Could you check a few things on this model? Use its own coordinates, in mm. A direction names the side the tool comes from. Round coordinates to 2 decimals unless told otherwise and drop trailing zeros. Loops run counter-clockwise (first coordinate to the right, second up) from the corner with the lowest first, then second, coordinate; pieces in that order, holes last. Notation, with made-up numbers: M -26,76.25 L -18,76.25 A19 ccw -18,113.25 Z; hole C 44.5,37.25 d3. An arc over 180 degrees is marked long. Return JSON: item names as keys, results as strings. Group by question number.
```python
from build123d import *

# Parameters (mm, degrees)
F2_DEPTH = 25


# Not quite as in the source:
# - a feature names something its author has since deleted; it is built from what else it names


with BuildPart() as f1:
    # F0 (on Front) → F1 (revolve)
    with BuildSketch(Plane.XZ):
        with BuildLine():
            Line((0, 9.9311807901), (0, 10.9311807901))
            Line((0, 10.9311807901), (-3.4236455734, 10.9311807901))
            ThreePointArc((-3.4236455734, 10.9311807901), (-3.9013040029, 10.5789726191), (-4.3789624324, 10.9311807901))
            Line((-4.3789624324, 10.9311807901), (-15.6210375676, 10.9311807901))
            ThreePointArc((-15.6210375676, 10.9311807901), (-16.0986959971, 10.5789726191), (-16.5763544266, 10.9311807901))
            Line((-16.5763544266, 10.9311807901), (-20, 10.9311807901))
            Line((-20, 10.9311807901), (-20, 9.9311807901))
            Line((-20, 9.9311807901), (-19, 9.9311807901))
            Line((-19, 9.9311807901), (-19, 7.4311807901))
            Line((-19, 7.4311807901), (-18.118519783, 7.4311807901))
            Line((-18.118519783, 7.4311807901), (-18.118519783, 3.4311807901))
            Line((-18.118519783, 3.4311807901), (-1.881480217, 3.4311807901))
            Line((-1.881480217, 3.4311807901), (-1.881480217, 7.4311807901))
            Line((-1.881480217, 7.4311807901), (-1, 7.4311807901))
            Line((-1, 7.4311807901), (-1, 9.9311807901))
            Line((-1, 9.9311807901), (0, 9.9311807901))
        make_face()
    revolve(axis=Axis((-10, 0, 3.4311807901), (-1, 0, 0)))

    # F2 (cut): a face of the model
    f2_faces = [f1.faces().sort_by_distance(p)[0] for p in [
        (-18.118519783, 0, 3.4311807901),
    ]]
    extrude(f2_faces, amount=-F2_DEPTH, mode=Mode.SUBTRACT)


solid = f1.part
```
1. I'm going to push flat-ended pins straight in: pin 1 Ø4 at (y, z) = (1, 5.5) entering from +X; pin 2 Ø6 at (x, y) = (-9.5, -5) entering from -Z; pin 3 Ø3 at (x, y) = (-15.5, -2) entering from -Z. Where does each tip first touch, or does it pass through?
2. We'd pull the mould along Y, two halves only. Please class faces 4 (the face through (-20, 7, 3)), 5 (the face through (-10.08, -2.87, 10.36)), 6 (the face through (-1, -4.2, 3.5)): +Y half, -Y half, draft (parallel to the pull), parting line (faces both ways), or undercut.
3. If we section it at A-A, the plane y = 0: Please give me the cut outline in (x, z).
4. On a 3-axis mill with a long thin cutter (end or side, diameter ignored), from which of +Z, -Z, +X, -X, +Y, -Y can I reach the whole of each face in a straight line? I mean faces 1 (the face through (0, 7, 3)), 2 (the face through (-19, -3, 0)), 3 (the face through (-0.493, -6.345, 2.022)). Say none if no direction works.
5. I need wall thicknesses on probe 1 along X at (y, z) = (6.25, 7.5); probe 2 along Z at (x, y) = (-11.25, 2); probe 3 along Z at (x, y) = (-17.25, -3.25). Which ranges of each line are inside material? Lowest first, please.
6. If we section it at B-B, the plane x = -13.5: Please give me the cut outline in (y, z), then the cut area to 3 significant figures.
Geometry results:
{
 "1": {"pin 1": "x = -1", "pin 2": "z = -3.8", "pin 3": "z = -4.05"},
 "2": {"face 4": "draft", "face 5": "parting line", "face 6": "undercut"},
 "3": {"outline": "M -20,-4.07 L -16.58,-4.07 A0.5 cw -15.62,-4.07 L -4.38,-4.07 A0.5 cw -3.42,-4.07 L 0,-4.07 L 0,-3.07 L -1,-3.07 L -1,-0.57 L -19,-0.57 L -19,-3.07 L -20,-3.07 Z; M -20,9.93 L -19,9.93 L -19,7.43 L -1,7.43 L -1,9.93 L 0,9.93 L 0,10.93 L -3.42,10.93 A0.5 cw -4.38,10.93 L -15.62,10.93 A0.5 cw -16.58,10.93 L -20,10.93 Z"},
 "4": {"face 1": "+Z, -Z, +X, +Y, -Y", "face 2": "-X", "face 3": "+X"},
 "5": {"probe 1": "-20 to -16.56, -15.64 to -4.36, -3.44 to 0", "probe 2": "-3.8 to -0.03, 6.9 to 10.66", "probe 3": "-3.33 to 1.1, 5.76 to 10.19"},
 "6": {"outline": "C 0,3.43 d15; hole C 0,3.43 d8", "area": "126 mm^2"}
}
